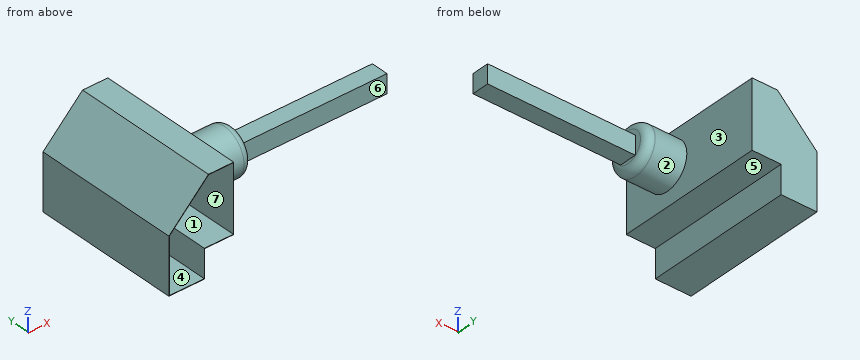
```python
from build123d import *

# Parameters (mm, degrees)
F1_DEPTH  = 95.1442476362
F4_SIZE   = 25.4
F5_T      = -0.254
F7_R      = 14.8113832011
F8_DEPTH  = 25.4
F9_W      = 11.0863484442
F9_H      = 11.992841959
F10_DEPTH = 94.742
F11_R     = 5.08


# Not quite as in the source:
# - the program builds the solid bodies; features that only make, move or delete a surface that nothing else refers to are left out


with BuildPart() as f1:
    # F0 (on Front) → F1 (new body)
    with BuildSketch(Plane.XZ):
        Polygon((-9.3385055661, 8.2524567842), (13.6685147882, 8.2524567842), (13.6685147882, 26.3094156981), (32.2877131402, 26.3094156981), (32.2877131402, 69.3843364716), (-9.3385055661, 69.3843364716), align=None)
    extrude(amount=F1_DEPTH)

    # F4
    f4_edges = [f1.edges().sort_by_distance(p)[0] for p in [
        (-9.338506, -47.572124, 69.384336),
    ]]
    chamfer(f4_edges, length=F4_SIZE)

    # F5
    f5_openings = [f1.faces().sort_by_distance(p)[0] for p in [
        (11.53567, -95.144248, 38.877913),
    ]]
    offset(amount=F5_T, openings=f5_openings, kind=Kind.INTERSECTION)

    # F7 (on face) → F8 (join)
    with BuildSketch(Plane.YZ.offset(32.2877131402)):
        with Locations((-64.1838386655, 50.4019707441)):
            Circle(F7_R)
    extrude(amount=F8_DEPTH)

    # F9 (on face) → F10 (join)
    with BuildSketch(Plane.YZ.offset(57.6877131402)):
        with Locations((-63.960975036, 48.7824268639)):
            Rectangle(F9_W, F9_H)
    extrude(amount=F10_DEPTH)

    # F11
    f11_edges = [f1.edges().sort_by_distance(p)[0] for p in [
        (57.687713, -78.995222, 50.401971),
    ]]
    fillet(f11_edges, radius=F11_R)


solid = f1.part
```
Input: part model. Units: mm. Frame: model coordinates. Face numbers are marked on the shaded views. A direction names the side the tool comes from. Give positions to 0.01 mm unless a question says otherwise; leave off trailing zeros. Order: outer loops, then holes, each group sorted by start corner. A loop starts at its lowest first (then second) coordinate and runs counter-clockwise, first axis right, second up. Notation, with made-up numbers: M 30.25,-14.5 L 56.25,-14.5 A19 cw 56.25,12.5 Z; hole C 1,71 d6. An arc over 180 degrees is marked long. Return JSON: item names as keys, results as strings.
Item 1: Pull-direction query (X, two-part tool) for the marked faces 1, 2, 3 and 4; classes: +X half, -X half, draft (parallel to the pull), parting line (faces both ways), or undercut.
Solutions:
{"face 1": "undercut", "face 2": "draft", "face 3": "+X half", "face 4": "undercut"}
Item 2: First-contact query: P1, Ø18, axis at x = 6, y = -45, coming from the +Z side; P2, Ø2, axis at x = 88, y = -60.5, coming from the +Z side; P3, Ø9.5, axis at x = 94, z = 48, coming from the +Y side. Flat tips, straight axial feed; report the tip coordinate or a pass-through.
Solutions:
{"P1": "z = 68.32", "P2": "z = 54.78", "P3": "y = -58.42"}
Item 3: Cut plane C-C (z = 19). Return loops of the section in (x, y).
Solutions:
{"outline": "M -9.34,-95.14 L -9.08,-95.14 L -9.08,-0.25 L 13.41,-0.25 L 13.41,-95.14 L 13.67,-95.14 L 13.67,0 L -9.34,0 Z"}
Item 4: Ray query, probe 1 along X at (y, z) = (-11.5, 42.5); probe 2 along Z at (x, y) = (27, -81); probe 3 along X at (y, z) = (-78, 22). Return the intervals inside material, ascending.
Solutions:
{"probe 1": "-9.34 to -9.08, 32.03 to 32.29", "probe 2": "26.31 to 26.56, 69.13 to 69.38", "probe 3": "-9.34 to -9.08, 13.41 to 13.67"}
Item 5: Cut plane B-B (z = 30). Return loops of the section in (x, y), then the cut area to 3 significant figures.
Solutions:
{"outline": "M -9.34,-95.14 L -9.08,-95.14 L -9.08,-0.25 L 32.03,-0.25 L 32.03,-95.14 L 32.29,-95.14 L 32.29,0 L -9.34,0 Z", "area": "58.8 mm^2"}
Item 6: Access query for the marked faces 5, 6 and 7. Directions: +Z, -Z, +X, -X, +Y, -Y. A direction counts if a zero-diameter tool reaches every point of the face in a straight line with its end or side. Return the directions, or none.
Solutions:
{"face 5": "-Z, +X, +Y, -Y", "face 6": "+Z, -Z, +X, -Y", "face 7": "-Y"}
Item 7: Cut plane D-D (x = 80). Return loops of the section in (y, z).
Solutions:
{"outline": "M -69.5,42.79 L -58.42,42.79 L -58.42,54.78 L -69.5,54.78 Z"}
Item 8: Cut plane A-A (y = -8.5). Return loops of the section in (x, z).
Solutions:
{"outline": "M -9.34,8.25 L 13.67,8.25 L 13.67,26.31 L 32.29,26.31 L 32.29,69.38 L 16.06,69.38 L -9.34,43.98 Z; hole M -9.08,8.51 L 13.41,8.51 L 13.41,26.56 L 32.03,26.56 L 32.03,69.13 L 16.17,69.13 L -9.08,43.88 Z"}
